Here's the drawing with two shaded views (mm, measured from the low corner). I have some questions. A direction names the side the tool comes from. Coordinates: 2 decimals unless noted, no trailing zeros. Loops run counter-clockwise (first coordinate to the right, second up) from the corner with the lowest first, then second, coordinate; pieces in that order, holes last. Notation, with made-up numbers: (84, 83) -> (137, 83) arc R18 cw to (137, 103) -> close; hole circle Ø1 at (6, 14.5). An arc over 180 degrees is marked (long way). Answer as a JSON object with one key per item and string values. Group by question number.
1) I want a section at D-D (x = 22.5). Write out the boundary of the cut face in (y, z).
2) I want a section at A-A (y = 63.5). Write out the boundary of the cut face in (x, z) (1 decimal).
3) I want a section at B-B (y = 97.5). Write out the boundary of the cut face in (x, z).
4) I'm going to push flat-ended pins straight in: pin 1 (3 mm diameter, centred on y = 35.5, z = 19, fed in from -X); pin 2 (2 mm diameter, centred on x = 13.5, y = 82, fed in from +Z). Where does each tip first touch, or does it pass through?
5) I need wall thicknesses on probe 1 along Y at (x, z) = (12.7, 0.8) (1 decimal); probe 2 along Z at (x, y) = (1.75, 63); probe 3 along X at (y, z) = (13, 5.25). Which ranges of each line are inside material? Lowest first, please. Write a range as [from, to].
6) I want a section at C-C (z = 9.25). Write out the boundary of the cut face in (x, y).
7) Which directions (+Z, -Z, +X, -X, +Y, -Y) give clear straight access to the entire face, cutting with the end or side of a thin tool? Please do the marked faces 1 and 2.
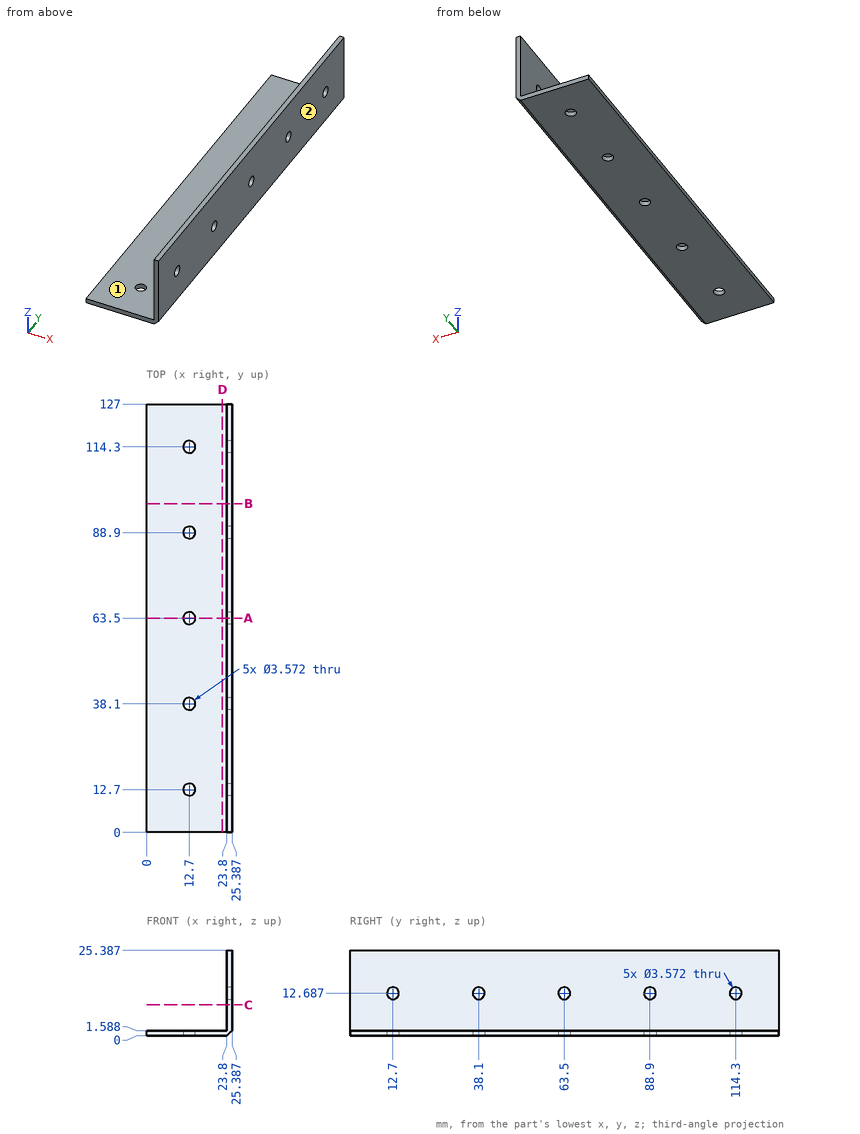
Determined:
{
 "1": {"outline": "(0, 0) -> (127, 0) -> (127, 1.59) -> (0, 1.59) -> close"},
 "2": {"outline": "(0, 0) -> (10.9, 0) -> (10.9, 1.6) -> (0, 1.6) -> close; (14.5, 0) -> (23.8, 0) -> (25.4, 1.6) -> (25.4, 10.9) -> (23.8, 10.9) -> (23.8, 1.6) -> (14.5, 1.6) -> close; (23.8, 14.5) -> (25.4, 14.5) -> (25.4, 25.4) -> (23.8, 25.4) -> close"},
 "3": {"outline": "(0, 0) -> (23.8, 0) -> (25.39, 1.59) -> (25.39, 25.39) -> (23.8, 25.39) -> (23.8, 1.59) -> (0, 1.59) -> close"},
 "4": {"pin 1": "x = 23.8", "pin 2": "z = 1.59"},
 "5": {"probe 1": "[0, 10.9], [14.5, 36.3], [39.9, 61.7], [65.3, 87.1], [90.7, 112.5], [116.1, 127]", "probe 2": "[0, 1.59]", "probe 3": "[23.8, 25.39]"},
 "6": {"outline": "(23.8, 0) -> (25.39, 0) -> (25.39, 127) -> (23.8, 127) -> close"},
 "7": {"face 1": "+Z, -X, +Y, -Y", "face 2": "+Z, -Z, +X, +Y, -Y"}
}
